Autodesk Inventor part; units mm, degrees
ref_plane "YZ Plane" through (0, 0, 0) normal (1, 0, 0) x (0, 1, 0)
ref_plane "XZ Plane" through (0, 0, 0) normal (0, 1, 0) x (-1, 0, 0)
ref_plane "XY Plane" through (0, 0, 0) normal (0, 0, 1) x (1, 0, 0)
sketch "スケッチ1" plane through (0, 0, 0) normal (0, 1, 0) x (-1, 0, 0)
  line L0 (0, 0) -> (-9, 0)
  line L1 (-9, 0) -> (-9, -9)
  line L2 (-9, -9) -> (0, -9)
  line L3 (0, -9) -> (0, 0)
  line L4 (-1.2, -1.2) -> (-7.8, -1.2)
  line L5 (-7.8, -1.2) -> (-7.8, -7.8)
  line L6 (-7.8, -7.8) -> (-1.2, -7.8)
  line L7 (-1.2, -7.8) -> (-1.2, -1.2)
  dimension "d0" = 9
  dimension "d1" = 9
  dimension "d2" = 6.6
  dimension "d3" = 6.6
  dimension "d4" = 1.2
  dimension "d5" = 1.2
extrude "押し出し1" add sketch "スケッチ1" along normal blind 113.5
sketch "スケッチ2" plane through (0, 0, 0) normal (0, 0, 1) x (1, 0, 0)
  line L0 (0, 0) -> (9, 0)
  line L1 (0, 0) -> (0, 113.5)
  point P0 (4.5, 29.5)
  point P1 (4.5, 13.5)
  dimension "d8" = 13.5
  dimension "d9" = 4.5
  dimension "d10" = 16
  dimension "d11" = 4.5
hole "穴1" at (4.5, 29.5, 0) at (4.5, 13.5, 0) direction (0, 0, -1) diameter 3 end through all
sketch "スケッチ3" plane through (0, 0, -9) normal (-1, 0, 0) x (0, 0, 1)
  line L0 (0, 0) -> (9, 0)
  line L1 (0, 0) -> (0, 113.5)
  point P0 (4.5, 4.5)
  point P1 (4.5, 74)
  dimension "d19" = 4.5
  dimension "d20" = 4.5
  dimension "d21" = 4.5
  dimension "d22" = 69.5
hole "穴2" at (0, 4.5, -4.5) at (0, 74, -4.5) direction (1, 0, 0) diameter 3 end through all
sketch "スケッチ4" plane through (0, 0, -9) normal (-1, 0, 0) x (0, 0, 1)
  line L0 (0, 113.5) -> (9, 113.5)
  line L1 (0, 0) -> (0, 113.5)
  point P0 (9, 0)
  point P1 (4.5, 100)
  dimension "d30" = 13.5
  dimension "d31" = 4.5
hole "穴3" at (0, 100, -4.5) direction (1, 0, 0) diameter 3 end through all
sketch "スケッチ5" plane through (9, 0, -9) normal (0, 0, -1) x (-1, 0, 0)
  line L0 (0, 113.5) -> (9, 113.5)
  line L1 (9, 0) -> (9, 113.5)
  point P0 (4.5, 109)
  dimension "d39" = 4.5
  dimension "d40" = 4.5
hole "穴4" at (4.5, 109, -9) direction (0, 0, 1) diameter 3 end through all
sketch "スケッチ6" plane through (9, 0, 0) normal (1, 0, 0) x (0, 0, -1)
  line L0 (0, 0) -> (0, 113.5)
  circle A0 centre (4.5, 4.5) radius 1.5
  point P0 (4.5, 38.5)
  dimension "d48" = 4.5
  dimension "d49" = 34
hole "穴5" at (9, 38.5, -4.5) direction (-1, 0, 0) diameter 3 end through all
properties part number "上下直動9x9_2" material "アルミニウム 6061"
Can you work these out from the model? Positions are in its coordinate system, mm. A direction names the side the tool comes from. Coordinates: 2 decimals unless noted, no trailing zeros. Order: outer loops, then holes, each group sorted by start corner. A loop starts at its lowest first (then second) coordinate and runs counter-clockwise, first axis right, second up.
1. For faces 1 (the face through (0.608, 98.513, -4.695)), 2 (the face through (5, 56, -7.8)), which set-ups out of +Z, -Z, +X, -X, +Y, -Y let a thin tool reach every point of the face, with its end or its side?
2. If we section it at B-B (y = 29.5): Please give me the cut outline in (x, z), then the cut area to 3 significant figures.
3. If we section it at C-C (z = -4.5): Give the number of separate pieces and of enclosed holes in the cut face, then the cut area to 3 significant figures.
4. Thinking about a two-plate mould opening in Y: for faces 3 (the face through (1, 0, -4)), 4 (the face through (7.8, 56, -4)), 5 (the face through (4.43, 15, -8.41)), which applies, +Y half, -Y half, draft (parallel to the pull), parting line (faces both ways), or undercut?
5. I'm going to push a flat-ended pin straight in: pin 1 (2.5 mm diameter, centred on x = 4.5, y = 29.5, fed in from -Z). Where does the tip first touch, or does it pass through?
6. If we section it at A-A (y = 69): Please give me the cut outline in (x, z).
7. I need wall thicknesses on line 1 (Y direction, x = 8.6, z = -4.5); line 2 (Y direction, x = 4.5, z = -0.65); line 3 (X direction, y = 106, z = -6.25). Which ranges of each line are inside material? Lowest first, please.
Entries:
1. face 1: +X, -X
1. face 2: +Y, -Y
2. outline: (0, -9) - (3, -9) - (3, -7.8) - (1.2, -7.8) - (1.2, -1.2) - (3, -1.2) - (3, 0) - (0, 0) - close; (6, -9) - (9, -9) - (9, 0) - (6, 0) - (6, -1.2) - (7.8, -1.2) - (7.8, -7.8) - (6, -7.8) - close
2. area: 30.2 mm2
3. separate pieces: 10
3. enclosed holes: 0
3. area: 244 mm2
4. face 3: -Y half
4. face 4: draft
4. face 5: undercut
5. pin 1: passes through
6. outline: (0, -9) - (9, -9) - (9, 0) - (0, 0) - close; hole (1.2, -7.8) - (7.8, -7.8) - (7.8, -1.2) - (1.2, -1.2) - close
7. line 1: y = 0 to 3, 6 to 37, 40 to 72.5, 75.5 to 98.5, 101.5 to 113.5
7. line 2: y = 0 to 12, 15 to 28, 31 to 107.5, 110.5 to 113.5
7. line 3: x = 0 to 1.2, 7.8 to 9
